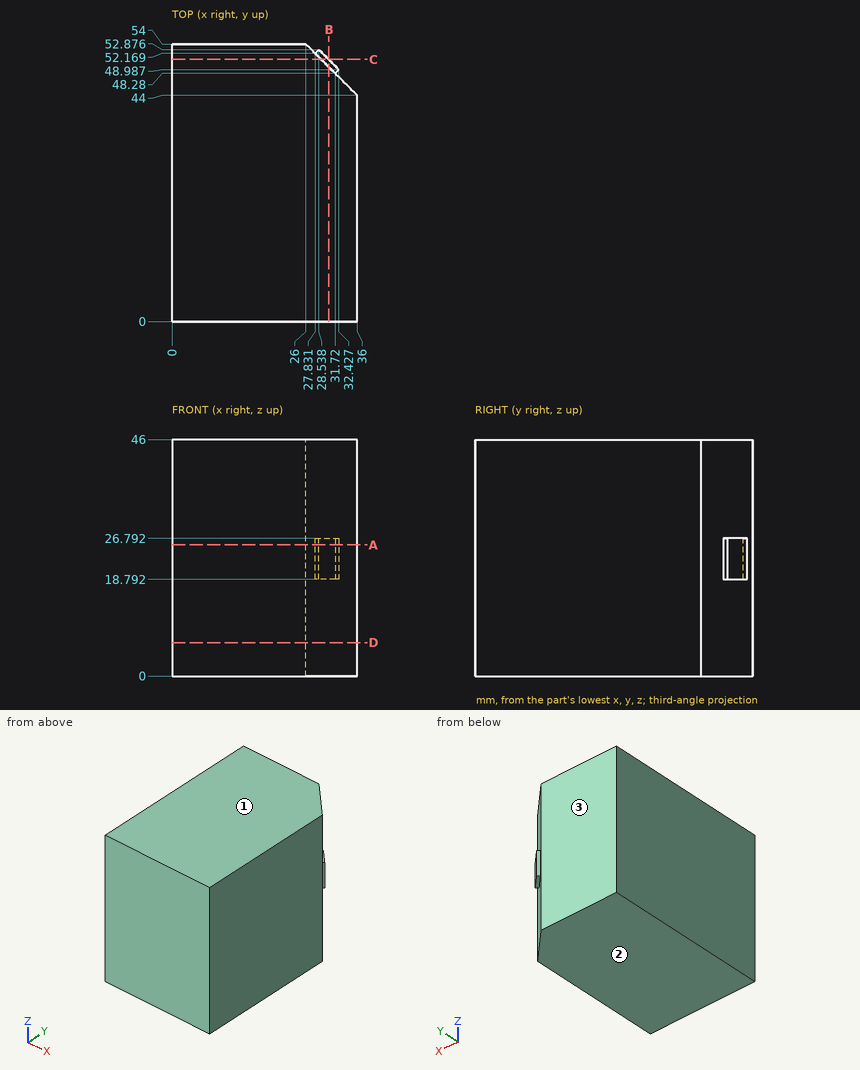
Input: dimensioned drawing with shaded views. Units: mm. Origin: part minimum x, y, z. Coordinates: 2 decimals unless noted, no trailing zeros. Order: outer loops, then holes, each group sorted by start corner. A loop starts at its lowest first (then second) coordinate and runs counter-clockwise, first axis right, second up.
(1) First-contact query: pin 1 (1.5 mm diameter, centred on x = 26.5, z = 23, fed in from -Y). Flat tip, straight axial feed; report the tip coordinate or a pass-through.
(2) Section query C-C (y = 51). Return the cut outline in (x, z).
(3) Section query B-B (x = 30.5). Return the cut outline in (y, z), plus the area to 3 significant figures.
(4) Section query A-A (z = 25.5). Return the cut outline in (x, y).
(5) Material intervals for probe 1 along X at (y, z) = (51.5, 11.5); probe 2 along X at (y, z) = (52.5, 40), sorted ascending.
(6) Draft query along Z for the marked faces 1, 2 and 3. Return one class per face: pulls with the +Z half, pulls with the -Z half, needs draft (parallel to the pull), parting line crosses it, or undercut.
(7) Section query D-D (z = 6.5). Return the cut outline in (x, y).
Solution:
1. pin 1: stops at y = 0
2. outline: (0, 0) - (29, 0) - (29, 18.79) - (30.41, 18.79) - (30.41, 26.79) - (29, 26.79) - (29, 46) - (0, 46) - close
3. outline: (0, 0) - (49.5, 0) - (49.5, 18.79) - (50.91, 18.79) - (50.91, 26.79) - (49.5, 26.79) - (49.5, 46) - (0, 46) - close
3. area: 2,290 mm2
4. outline: (0, 0) - (36, 0) - (36, 44) - (31.72, 48.28) - (32.43, 48.99) - (28.54, 52.88) - (27.83, 52.17) - (26, 54) - (0, 54) - close
5. probe 1: x = 0 to 28.5
5. probe 2: x = 0 to 27.5
6. face 1: pulls with the +Z half
6. face 2: pulls with the -Z half
6. face 3: needs draft
7. outline: (0, 0) - (36, 0) - (36, 44) - (26, 54) - (0, 54) - close
